Here's how the part is built. I have some questions about the finished solid (model axes, mm). Face numbers are marked on the shaded views. A direction names the side the tool comes from. Round coordinates to 2 decimals unless told otherwise and drop trailing zeros. Order: outer loops, then holes, each group sorted by start corner. A loop starts at its lowest first (then second) coordinate and runs counter-clockwise, first axis right, second up. Notation, with made-up numbers: (-34, 48) - (-3, 48) arc R12 ccw to (-3, 59) - close; hole circle Ø9 at (60.25, 36). An arc over 180 degrees is marked (long way). One line per item, written item: value.
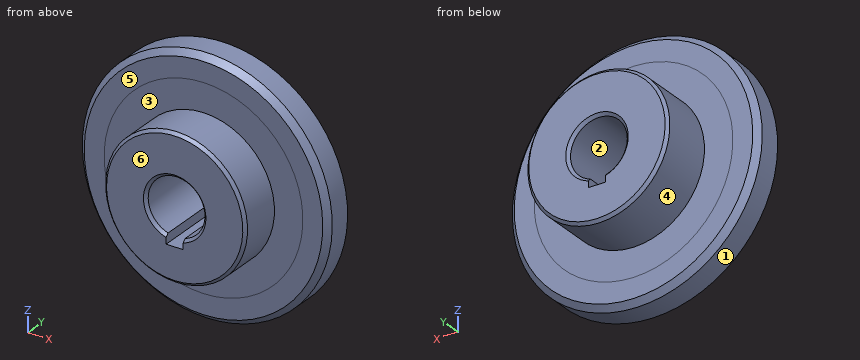
from build123d import *

# Parameters (mm, degrees)
SKETCH_1_W          = 17.5
SKETCH_1_H          = 6
SKETCH_5_W          = 12.5
SKETCH_5_H          = 23
SKETCH_10_R         = 5
CUT_EXTRUDE_3_DEPTH = 39.691197966
CHAMFER_3_SIZE      = 0.5
SKETCH_2_W          = 3
SKETCH_2_H          = 54.842712326
CUT_EXTRUDE_1_DEPTH = 6.4


with BuildPart() as part:
    # Sketch 1 → Revolve 729 (revolve)
    with BuildSketch(Plane.XY, mode=Mode.PRIVATE) as revolve_729_sk:
        with Locations((8.75, 3)):
            Rectangle(SKETCH_1_W, SKETCH_1_H)
    revolve(revolve_729_sk.sketch.rotate(Axis((0, 0, 0), (0, 1, 0)), 90), axis=Axis((0, 0, 0), (0, 1, 0)))

    # Sketch 3 → Revolve 1176 (revolve)
    with BuildSketch(Plane.XY, mode=Mode.PRIVATE) as revolve_1176_sk:
        Polygon((17.4999, -0.0001), (17.4999, 6.0001), (21.000041421, 6.0001), (22.0001, 5.000041421), (22.0001, 0.999958579), (21.000041421, -0.0001), align=None)
        Polygon((17.5, 0), (17.5, 6), (21, 6), (22, 5), (22, 1), (21, 0), align=None, mode=Mode.SUBTRACT)
    revolve(revolve_1176_sk.sketch.rotate(Axis((0, 0, 0), (0, 1, 0)), 90), axis=Axis((0, 0, 0), (0, 1, 0)))

    # Sketch 5 → Revolve 2677 (revolve)
    with BuildSketch(Plane.XY, mode=Mode.PRIVATE) as revolve_2677_sk:
        with Locations((6.25, 4)):
            Rectangle(SKETCH_5_W, SKETCH_5_H)
    revolve(revolve_2677_sk.sketch.rotate(Axis((0, -50, 0), (0, 1, 0)), 90), axis=Axis((0, -50, 0), (0, 1, 0)))

    # Sketch 10 → Cut-Extrude 3 (cut, through all)
    with BuildSketch(Plane(origin=(0, 15.5, 0), x_dir=(1, 0, 0), z_dir=(0, 1, 0))):
        with Locations(Location((0, 0, 0), (0, 0, 270))):
            Circle(SKETCH_10_R)
    extrude(amount=-CUT_EXTRUDE_3_DEPTH, mode=Mode.SUBTRACT)

    # Chamfer 3
    chamfer_3_edges = [part.edges().sort_by_distance(p)[0] for p in [
        (0, -7.5, 12.5),
        (0, 15.5, 12.5),
        (0, -7.5, -5),
        (0, 15.5, -5),
    ]]
    chamfer(chamfer_3_edges, length=CHAMFER_3_SIZE)

    # Sketch 2 → Cut-Extrude 1 (cut)
    with BuildSketch(Plane.XY):
        Rectangle(SKETCH_2_W, SKETCH_2_H)
    extrude(amount=-CUT_EXTRUDE_1_DEPTH, mode=Mode.SUBTRACT)


solid = part.part
Q1. We'd pull the mould along Z, two halves only. Please class the marked faces 1, 2 and 3: released by +Z, released by -Z, zero draft, split by the parting line, or undercut.
Results list:
face 1: split by the parting line
face 2: undercut
face 3: zero draft
Q2. If we section it at C-C, the plane y = -3.75: Please give me the cut outline in (x, z).
Results list:
outline: circle Ø25 at (0, 0); hole (-1.5, -6.4) - (1.5, -6.4) - (1.5, -4.77) arc R5 ccw (long way) to (-1.5, -4.77) - close
Q3. Which directions (+Z, -Z, +X, -X, +Y, -Y) give clear straight access to the entire face, cutting with the end or side of a thin tool? Please do the marked faces 4, 5 and 6.
Results list:
face 4: +Y
face 5: -Y
face 6: +Z, -Z, +X, -X, -Y
Q4. Will these pins go through, and if not, where does the flat tip stop? pin 1 (0.8 mm diameter, centred on y = 0.5, z = -6, fed in from +X); pin 2 (1 mm diameter, centred on x = -4, y = -3.5, fed in from -Z); pin 3 (3 mm diameter, centred on y = -2, z = 6.5, fed in from +X).
Results list:
pin 1: x = 21.08
pin 2: z = -12
pin 3: x = 11.46
Q5. If we section it at A-A, the plane x = 0: Give the number of separate pieces and of enclosed holes in the cut face, then the cut area to 3 significant figures.
Results list:
separate pieces: 2
enclosed holes: 2
area: 372 mm²
Q6. If I drill on line 1 along X through (y, z) = (-3.25, 0); line 2 along Y through (x, z) = (-15.5, -3); line 3 along Z through (x, y) = (9, 8.5), over which ranges is the centre line in solid material (lowest first)?
Results list:
line 1: -12.5 to -5, 5 to 12.5
line 2: 0 to 6
line 3: -8.67 to 8.67
